```python
from build123d import *

# Parameters (mm, degrees)
SKETCH_1_W          = 80
SKETCH_1_H          = 60
SKETCH_1_R          = 2.15
EXTRUDE_1_DEPTH     = 5
SKETCH_2_R          = 2.15
CUT_EXTRUDE_1_DEPTH = 68.134361545
SKETCH_3_R          = 2.15
CUT_EXTRUDE_2_DEPTH = 68.134361545
CUT_EXTRUDE_3_DEPTH = 68.134361545
FILLET_1_R          = 5
SKETCH_5_R          = 2.15
CUT_EXTRUDE_4_DEPTH = 68.134361545
FILLET_2_R          = 5
EXTRUDE_2_DEPTH     = 5
FILLET_3_R          = 10


with BuildPart() as part:
    # ｽｹｯﾁ1 → ﾎﾞｽ - 押し出し1 (new body)
    with BuildSketch(Plane.XY):
        with Locations((-19.85, 0)):
            Rectangle(SKETCH_1_W, SKETCH_1_H)
        with Locations((-5, -24.75)):
            Circle(SKETCH_1_R, mode=Mode.SUBTRACT)
        with Locations((5, -24.75)):
            Circle(SKETCH_1_R, mode=Mode.SUBTRACT)
        Polygon((0.65, -20.15), (0.65, -27.15), (-0.65, -27.15), (-0.65, -20.15), (-10.15, -20.15), (-10.15, 20.15), (-0.65, 20.15), (-0.65, 27.15), (0.65, 27.15), (0.65, 20.15), (10.15, 20.15), (10.15, -20.15), align=None, mode=Mode.SUBTRACT)
        with Locations((-5, 24.75)):
            Circle(SKETCH_1_R, mode=Mode.SUBTRACT)
        with Locations((5, 24.75)):
            Circle(SKETCH_1_R, mode=Mode.SUBTRACT)
    extrude(amount=EXTRUDE_1_DEPTH)

    # ｽｹｯﾁ2 → ｶｯﾄ - 押し出し1 (cut, through all)
    with BuildSketch(Plane.XY.offset(5)):
        with Locations((-54.85, 10)):
            Circle(SKETCH_2_R)
        with Locations(Location((-54.85, -10, 0), (0, 0, 180))):
            Circle(SKETCH_2_R)
        with Locations((-34.85, 10)):
            Circle(SKETCH_2_R)
        with Locations(Location((-34.85, -10, 0), (0, 0, 180))):
            Circle(SKETCH_2_R)
    extrude(amount=-CUT_EXTRUDE_1_DEPTH, mode=Mode.SUBTRACT)

    # ｽｹｯﾁ3 → ｶｯﾄ - 押し出し2 (cut, through all)
    with BuildSketch(Plane.XY.offset(5)):
        with Locations((15.15, 25)):
            Circle(SKETCH_3_R)
        with BuildLine():
            ThreePointArc((15.15, 30), (18.685533906, 28.535533906), (20.15, 25))
            Line((20.15, 25), (20.15, 30))
            Line((20.15, 30), (15.15, 30))
        make_face()
    extrude(amount=-CUT_EXTRUDE_2_DEPTH, mode=Mode.SUBTRACT)

    # ｽｹｯﾁ4 → ｶｯﾄ - 押し出し3 (cut, through all)
    with BuildSketch(Plane.XY.offset(5)):
        Polygon((-59.85, 30), (-59.85, 15.001700458), (-29.85, 30), align=None)
        Polygon((-29.85, -30), (-59.85, -15.001700458), (-59.85, -30), align=None)
    extrude(amount=-CUT_EXTRUDE_3_DEPTH, mode=Mode.SUBTRACT)

    # ﾌｨﾚｯﾄ1
    fillet_1_edges = [part.edges().sort_by_distance(p)[0] for p in [
        (20.15, -30, 2.5),
    ]]
    fillet(fillet_1_edges, radius=FILLET_1_R)

    # ｽｹｯﾁ5 → ｶｯﾄ - 押し出し4 (cut, through all)
    with BuildSketch(Plane.XY.offset(5)):
        with Locations((-28.669779796, -25)):
            Circle(SKETCH_5_R)
    extrude(amount=-CUT_EXTRUDE_4_DEPTH, mode=Mode.SUBTRACT)

    # ﾌｨﾚｯﾄ2
    fillet_2_edges = [part.edges().sort_by_distance(p)[0] for p in [
        (-59.85, 15.001700458, 2.5),
        (-29.85, 30, 2.5),
        (-59.85, -15.001700458, 2.5),
        (-29.85, -30, 2.5),
    ]]
    fillet(fillet_2_edges, radius=FILLET_2_R)

    # ｽｹｯﾁ6 → ﾎﾞｽ - 押し出し2 (add)
    with BuildSketch(Plane.XY.offset(5)):
        with BuildLine():
            ThreePointArc((2.5, 30), (0, 32.5), (-2.5, 30))
            Line((-2.5, 30), (2.5, 30))
        make_face()
        with BuildLine():
            Line((2.5, 30), (-2.5, 30))
            ThreePointArc((-2.5, 30), (0, 27.5), (2.5, 30))
        make_face()
        with BuildLine():
            ThreePointArc((2.5, -30), (0, -27.5), (-2.5, -30))
            Line((-2.5, -30), (2.5, -30))
        make_face()
        with BuildLine():
            Line((2.5, -30), (-2.5, -30))
            ThreePointArc((-2.5, -30), (0, -32.5), (2.5, -30))
        make_face()
    extrude(amount=-EXTRUDE_2_DEPTH)

    # ﾌｨﾚｯﾄ3
    fillet_3_edges = [part.edges().sort_by_distance(p)[0] for p in [
        (2.5, 30, 2.5),
        (-2.5, 30, 2.5),
        (2.5, -30, 2.5),
        (-2.5, -30, 2.5),
    ]]
    fillet(fillet_3_edges, radius=FILLET_3_R)


solid = part.part
```
Input: part model. Units: mm. Frame: model coordinates. A direction names the side the tool comes from. Give positions to 0.01 mm unless a question says otherwise; leave off trailing zeros. Order: outer loops, then holes, each group sorted by start corner. A loop starts at its lowest first (then second) coordinate and runs counter-clockwise, first axis right, second up. Notation, with made-up numbers: M -9,-21 L 20,-21 A27 cw 20,9 Z; hole C 65.25,73.25 d5. An arc over 180 degrees is marked long. One line per question, with ' | ' between items.
1) Contact query for flat-ended pins moving along their axis: P1, Ø6, axis at x = 9, y = -8.5, coming from the -Z side; P2, Ø2.5, axis at x = -20, z = 2.5, coming from the -Y side; P3, Ø2, axis at x = -47.5, z = 1, coming from the +Y side; P4, Ø2.5, axis at x = -3, z = 2, coming from the -Y side. Output: stop coordinate, or through.
Filled in:
P1: stops at z = 0 | P2: stops at y = -30 | P3: stops at y = 21.68 | P4: stops at y = -31.82
2) Section A-A on y = 1.5. Output: boundary loops of the cut face in (x, z).
Filled in:
outline: M -59.85,0 L -10.15,0 L -10.15,5 L -59.85,5 Z; M 10.15,0 L 20.15,0 L 20.15,5 L 10.15,5 Z
3) Section D-D on z = 2.95. State how many separate pieces and enclosed holes the cut face has, and give its area (3 significant figures).
Filled in:
separate pieces: 1 | enclosed holes: 11 | area: 3,380 mm2
4) Ray query, L1, parallel to X at y = -10, z = 1.5; L2, parallel to X at y = 5, z = 4.65; L3, parallel to Y at x = -4, z = 3.8. Return the intervals inside material, ascending.
Filled in:
L1: x = -59.85 to -57, -52.7 to -37, -32.7 to -10.15, 10.15 to 20.15 | L2: x = -59.85 to -10.15, 10.15 to 20.15 | L3: y = -30.63 to -26.65, -22.85 to -20.15, 20.15 to 22.85, 26.65 to 30.63
5) Section C-C on x = -34.85. Output: boundary loops of the cut face in (y, z), and give its area (3 significant figures).
Filled in:
outline: M -27.5,0 L -12.15,0 L -12.15,5 L -27.5,5 Z; M -7.85,0 L 7.85,0 L 7.85,5 L -7.85,5 Z; M 12.15,0 L 27.5,0 L 27.5,5 L 12.15,5 Z | area: 232 mm2
6) Draft query along X for faces 5 (the face through (-59.083, 14.573, 2.465)), 6 (the face through (20.15, 0, 2)), 7 (the face through (-55.84, -8.09, 2.54)). Return one class per face: pulls with the +X half, pulls with the -X half, needs draft (parallel to the pull), parting line crosses it, or undercut.
Filled in:
face 5: pulls with the -X half | face 6: pulls with the +X half | face 7: undercut
7) Access query for faces 1 (the face through (5, -20.15, 2)), 2 (the face through (-18, 30, 2)), 3 (the face through (11, 30, 2)), 4 (the face through (-59.083, -14.573, 2.465)). Directions: +Z, -Z, +X, -X, +Y, -Y. A direction counts if a zero-diameter tool reaches every point of the face in a straight line with its end or side. Return the directions, or none.
Filled in:
face 1: +Z, -Z | face 2: +Z, -Z, -X, +Y | face 3: +Z, -Z, +X, +Y | face 4: +Z, -Z, -X, -Y
8) Section B-B on x = 8.5. Output: boundary loops of the cut face in (y, z), and give its area (3 significant figures).
Filled in:
outline: M -30,0 L -20.15,0 L -20.15,5 L -30,5 Z; M 20.15,0 L 30,0 L 30,5 L 20.15,5 Z | area: 98.5 mm2
